```python
from build123d import *

# Parameters (mm, degrees)
BOX_W           = 56
BOX_H           = 22
BOX_DEPTH       = 26
SKETCH_R        = 8
POCKET_DEPTH    = 56.001
SKETCH001_R     = 3.5
POCKET001_DEPTH = 23
SKETCH002_R     = 1.8
POCKET002_DEPTH = 5
SKETCH003_R     = 1.8
POCKET003_DEPTH = 22.001
SKETCH004_W     = 2
SKETCH004_H     = 11.298807
SKETCH004_W_2   = 3
SKETCH004_H_2   = 8
POCKET004_DEPTH = 56.001
FILLET_R        = 1


with BuildPart() as part:
    # Box → Box (new body)
    with BuildSketch(Plane.XY):
        with Locations((28, 11)):
            Rectangle(BOX_W, BOX_H)
    extrude(amount=BOX_DEPTH)

    # Sketch → Pocket (cut, through all)
    with BuildSketch(Plane.YZ.offset(56)):
        with Locations((11, 12.7)):
            Circle(SKETCH_R)
    extrude(amount=-POCKET_DEPTH, mode=Mode.SUBTRACT)

    # Sketch001 → Pocket001 (cut)
    with BuildSketch(Plane.XY.offset(26)):
        with Locations((10, 11)):
            Circle(SKETCH001_R)
        with Locations((46, 11)):
            Circle(SKETCH001_R)
    extrude(amount=-POCKET001_DEPTH, mode=Mode.SUBTRACT)

    # Sketch002 → Pocket002 (cut)
    with BuildSketch(Plane(origin=(0, 0, 0), x_dir=(1, 0, 0), z_dir=(0, 0, -1))):
        with Locations((10, -11)):
            Circle(SKETCH002_R)
        with Locations((46, -11)):
            Circle(SKETCH002_R)
    extrude(amount=-POCKET002_DEPTH, mode=Mode.SUBTRACT)

    # Sketch003 → Pocket003 (cut, through all)
    with BuildSketch(Plane(origin=(0, 22, 0), x_dir=(-1, 0, 0), z_dir=(0, 1, 0))):
        with Locations((-35.5, 22.5)):
            Circle(SKETCH003_R)
        with Locations((-20.5, 22.5)):
            Circle(SKETCH003_R)
    extrude(amount=-POCKET003_DEPTH, mode=Mode.SUBTRACT)

    # Sketch004 → Pocket004 (cut, through all)
    with BuildSketch(Plane.YZ.offset(56)):
        with Locations((11, 23.747477)):
            Rectangle(SKETCH004_W, SKETCH004_H)
        with Locations((1.5, 22)):
            Rectangle(SKETCH004_W_2, SKETCH004_H_2)
        with Locations((20.5, 22)):
            Rectangle(SKETCH004_W_2, SKETCH004_H_2)
    extrude(amount=-POCKET004_DEPTH, mode=Mode.SUBTRACT)

    # Fillet
    fillet_edges = [part.edges().sort_by_distance(p)[0] for p in [
        (28, 0, 18),
        (28, 3, 18),
        (28, 3, 26),
        (28, 19, 26),
        (28, 19, 18),
        (28, 22, 18),
    ]]
    fillet(fillet_edges, radius=FILLET_R)


solid = part.part
```
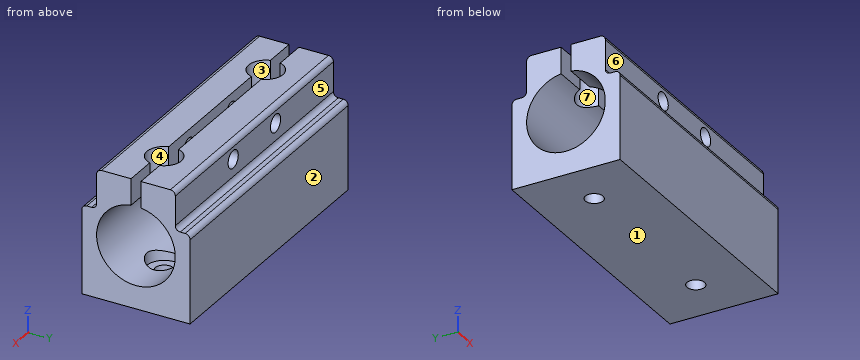
Part model, mm, in its own coordinate system. Face numbers are marked on the shaded views. A direction names the side the tool comes from. Coordinates: 2 decimals unless noted, no trailing zeros. Order: outer loops, then holes, each group sorted by start corner. A loop starts at its lowest first (then second) coordinate and runs counter-clockwise, first axis right, second up. Notation, with made-up numbers: (0, 79.25) - (20, 79.25) arc R28 cw to (20, 109.25) - close; hole circle Ø11 at (48, 42). An arc over 180 degrees is marked (long way). Return JSON: item names as keys, results as strings. Group by question number.
Item 1: Pin check, flat tips, straight feed: pin 1 (6 mm diameter, centred on x = 52, z = 23, fed in from +Y); pin 2 (4.5 mm diameter, centred on x = 31.5, z = 22.5, fed in from -Y); pin 3 (5 mm diameter, centred on x = 32.5, z = 21, fed in from +Y); pin 4 (3 mm diameter, centred on x = 35.5, z = 22.5, fed in from +Y). Stop position of each tip, or through.
Item 2: Cut at A-A (y = 11). List the corners of the cut face in (x, z).
Item 3: Pull direction Y, two halves, no side cores. Call the marked faces 1, 2, 3 and 4: pulls with the +Y half, pulls with the -Y half, needs draft (parallel to the pull), parting line crosses it, or undercut.
Item 4: Cut at B-B (z = 22.5). State how many separate pieces and enclosed holes the cut face has, plus the area to 3 significant figures.
Item 5: Which spindle directions (+Z, -Z, +X, -X, +Y, -Y) get a long thin tool onto all of the face, cutting with end or side? Do the marked faces 5, 6 and 7. Say none if no direction does.
Item 6: Cut at D-D (z = 12.7). List the corners of the cut face in (x, y).
Item 7: Drill centre lines: probe 1 along X at (y, z) = (11, 0.9); probe 2 along Y at (x, z) = (32.5, 24.5); probe 3 along X at (y, z) = (6.25, 23.5). Where is each one in solid material? Low to high. Write a range as from..to.
Item 8: Cut at C-C (x = 10). List the corners of the cut face in (y, z), plus the area to 3 significant figures.
Check values:
{
 "1": {"pin 1": "stops at y = 19", "pin 2": "stops at y = 3", "pin 3": "stops at y = 19.13", "pin 4": "passes through"},
 "2": {"outline": "(0, 0) - (8.2, 0) - (8.2, 3) - (6.5, 3) - (6.5, 4.7) - (0, 4.7) - close; (11.8, 0) - (44.2, 0) - (44.2, 3) - (42.5, 3) - (42.5, 4.7) - (13.5, 4.7) - (13.5, 3) - (11.8, 3) - close; (47.8, 0) - (56, 0) - (56, 4.7) - (49.5, 4.7) - (49.5, 3) - (47.8, 3) - close"},
 "3": {"face 1": "needs draft", "face 2": "pulls with the +Y half", "face 3": "undercut", "face 4": "undercut"},
 "4": {"separate pieces": "6", "enclosed holes": "0", "area": "634 mm2"},
 "5": {"face 5": "+Z, +X, -X, +Y", "face 6": "+Z, +X, -X, -Y", "face 7": "+Z"},
 "6": {"outline": "(0, 0) - (56, 0) - (56, 3) - (0, 3) - close; (0, 19) - (56, 19) - (56, 22) - (0, 22) - close"},
 "7": {"probe 1": "x = 0..8.2, 11.8..44.2, 47.8..56", "probe 2": "y = 3..10, 12..19", "probe 3": "x = 0..19, 22..34, 37..56"},
 "8": {"outline": "(0, 0) - (9.2, 0) - (9.2, 3) - (7.5, 3) - (7.5, 5.51) arc R8 cw to (7.5, 19.89) - (7.5, 26) - (4, 26) arc R1 ccw to (3, 25) - (3, 19) arc R1 cw to (2, 18) - (1, 18) arc R1 ccw to (0, 17) - close; (12.8, 0) - (22, 0) - (22, 17) arc R1 ccw to (21, 18) - (20, 18) arc R1 cw to (19, 19) - (19, 25) arc R1 ccw to (18, 26) - (14.5, 26) - (14.5, 19.89) arc R8 cw to (14.5, 5.51) - (14.5, 3) - (12.8, 3) - close", "area": "259 mm2"}
}
